Check sheet for the modelled part. Datum: model origin and axes. Units: mm. A direction names the side the tool comes from. Coordinates: 2 decimals unless noted, no trailing zeros. Loops run counter-clockwise (first coordinate to the right, second up) from the corner with the lowest first, then second, coordinate; pieces in that order, holes last. Notation, with made-up numbers: M 10.25,65.25 L 14.25,65.25 A14 ccw 14.25,72.25 Z; hole C 64,67.5 d2. An arc over 180 degrees is marked long. Write each question's results on one line, items separated by ' | '. Start each with the question number.
from build123d import *

# Parameters (mm, degrees)
F0_W      = 95
F0_H      = 138.5
F1_DEPTH  = 2.5
F2_W      = 95
F2_H      = 138.5
F2_W_2    = 62
F2_H_2    = 123
F3_DEPTH  = 8.5
F4_W      = 95
F4_H      = 138.5
F5_DEPTH  = 23.5
F6_W      = 62
F6_H      = 123
F7_DEPTH  = 23.501
F8_W      = 95
F8_H      = 138.5
F8_W_2    = 90
F8_H_2    = 133.5
F9_DEPTH  = 17.5
F11_ANGLE = 180
F13_ANGLE = 180
F14_W     = 0.75
F14_H     = 7.75
F16_W     = 0.75
F16_H     = 7.75


with BuildPart() as f1:
    # F0 (on Top) → F1 (new body)
    with BuildSketch(Plane.XY):
        Rectangle(F0_W, F0_H)
    extrude(amount=F1_DEPTH)

    # F2 (on face) → F3 (join)
    with BuildSketch(Plane.XY.offset(2.5)):
        Rectangle(F2_W, F2_H)
        Rectangle(F2_W_2, F2_H_2, mode=Mode.SUBTRACT)
    extrude(amount=F3_DEPTH)

    # F4 (on face) → F5 (join)
    with BuildSketch(Plane.XY.offset(11)):
        with BuildLine():
            ThreePointArc((-22.25, 22.25), (-6.516874, 28.766874), (0, 44.5))
            ThreePointArc((0, 44.5), (-37.983126, 60.233126), (-22.25, 22.25))
        make_face()
        with BuildLine():
            ThreePointArc((44.5, 44.5), (22.25, 66.75), (0, 44.5))
            ThreePointArc((0, 44.5), (6.516874, 28.766874), (22.25, 22.25))
            ThreePointArc((22.25, 22.25), (37.983126, 28.766874), (44.5, 44.5))
        make_face()
        with BuildLine():
            ThreePointArc((0, 0), (-6.516874, 15.733126), (-22.25, 22.25))
            ThreePointArc((-22.25, 22.25), (-44.5, 0), (-22.25, -22.25))
            ThreePointArc((-22.25, -22.25), (-6.516874, -15.733126), (0, 0))
        make_face()
        with BuildLine():
            ThreePointArc((44.5, 0), (37.983126, 15.733126), (22.25, 22.25))
            ThreePointArc((22.25, 22.25), (6.516874, 15.733126), (0, 0))
            ThreePointArc((0, 0), (6.516874, -15.733126), (22.25, -22.25))
            ThreePointArc((22.25, -22.25), (37.983126, -15.733126), (44.5, 0))
        make_face()
        with BuildLine():
            ThreePointArc((0, -44.5), (-6.516874, -28.766874), (-22.25, -22.25))
            ThreePointArc((-22.25, -22.25), (-37.983126, -60.233126), (0, -44.5))
        make_face()
        with BuildLine():
            ThreePointArc((44.5, -44.5), (37.983126, -28.766874), (22.25, -22.25))
            ThreePointArc((22.25, -22.25), (6.516874, -28.766874), (0, -44.5))
            ThreePointArc((0, -44.5), (22.25, -66.75), (44.5, -44.5))
        make_face()
        Rectangle(F4_W, F4_H)
        with BuildLine():
            ThreePointArc((-22.25, 22.25), (-37.983126, 60.233126), (0, 44.5))
            ThreePointArc((0, 44.5), (22.25, 66.75), (44.5, 44.5))
            ThreePointArc((44.5, 44.5), (37.983126, 28.766874), (22.25, 22.25))
            ThreePointArc((22.25, 22.25), (37.983126, 15.733126), (44.5, 0))
            ThreePointArc((44.5, 0), (37.983126, -15.733126), (22.25, -22.25))
            ThreePointArc((22.25, -22.25), (37.983126, -28.766874), (44.5, -44.5))
            ThreePointArc((44.5, -44.5), (22.25, -66.75), (0, -44.5))
            ThreePointArc((0, -44.5), (-37.983126, -60.233126), (-22.25, -22.25))
            ThreePointArc((-22.25, -22.25), (-44.5, 0), (-22.25, 22.25))
        make_face(mode=Mode.SUBTRACT)
    extrude(amount=F5_DEPTH)

    # F6 (on face) → F7 (cut, through all)
    with BuildSketch(Plane.XY.offset(11)):
        Rectangle(F6_W, F6_H)
    extrude(amount=F7_DEPTH, mode=Mode.SUBTRACT)

    # F8 (on face) → F9 (join)
    with BuildSketch(Plane.XY.offset(34.5)):
        Rectangle(F8_W, F8_H)
        Rectangle(F8_W_2, F8_H_2, mode=Mode.SUBTRACT)
    extrude(amount=F9_DEPTH)

    # F10 (on face) → F11 (revolve)
    with BuildSketch(Plane.YZ.offset(-45)):
        with BuildLine():
            Line((0, 36.5), (0, 34.5))
            ThreePointArc((0, 34.5), (1.414214, 35.085786), (2, 36.5))
            Line((2, 36.5), (2, 50))
            ThreePointArc((2, 50), (1.414214, 51.414214), (0, 52))
            Line((0, 52), (0, 50))
            Line((0, 50), (0, 36.5))
        make_face()
    revolve(axis=Axis((-45, 0, 43.25), (0, 0, -1)), revolution_arc=F11_ANGLE)

    # F12 (on face) → F13 (revolve)
    with BuildSketch(Plane(origin=(45, 0, 0), x_dir=(0, -1, 0), z_dir=(-1, 0, 0))):
        with BuildLine():
            ThreePointArc((-2, 36.5), (-1.414214, 35.085786), (0, 34.5))
            Line((0, 34.5), (0, 36.5))
            Line((0, 36.5), (0, 50))
            Line((0, 50), (-2, 50))
            Line((-2, 50), (-2, 36.5))
        make_face()
        with BuildLine():
            Line((-2, 50), (0, 50))
            Line((0, 50), (0, 52))
            ThreePointArc((0, 52), (-1.414214, 51.414214), (-2, 50))
        make_face()
    revolve(axis=Axis((45, 0, 43.25), (0, 0, 1)), revolution_arc=F13_ANGLE)

    # F14 (on face) → F15 (revolve)
    with BuildSketch(Plane.YZ.offset(-31)):
        with BuildLine():
            ThreePointArc((0.75, 10.25), (0.53033, 10.78033), (0, 11))
            Line((0, 11), (0, 10.25))
            Line((0, 10.25), (0.75, 10.25))
        make_face()
        with Locations((0.375, 6.375)):
            Rectangle(F14_W, F14_H)
    revolve(axis=Axis((-31, 0, 6.75), (0, 0, -1)))

    # F16 (on face) → F17 (revolve)
    with BuildSketch(Plane(origin=(31, 0, 0), x_dir=(0, -1, 0), z_dir=(-1, 0, 0))):
        with Locations((-0.375, 6.375)):
            Rectangle(F16_W, F16_H)
        with BuildLine():
            Line((-0.75, 10.25), (0, 10.25))
            Line((0, 10.25), (0, 11))
            ThreePointArc((0, 11), (-0.53033, 10.78033), (-0.75, 10.25))
        make_face()
    revolve(axis=Axis((31, 0, 6.75), (0, 0, 1)))


solid = f1.part
1) Set-up check for faces 5 (the flat face through (34, 49, 11)), 6 (the flat face through (47.5, -1, 26)): record each of +Z, -Z, +X, -X, +Y, -Y from which the full face is reachable in a straight line by a thin tool's end or side.
2) Section check A-A (z = 40). Enter the section's corners in (x, y), then the cut area to 3 significant figures.
3) Section check B-B (x = -36.5). Enter the section's corners in (y, z).
4) Gauge pin test, flat ends, axial feed: P1, Ø7, axis at x = -35, y = -10, coming from the +Z side; P2, Ø10, axis at x = -35, y = 22.5, coming from the +Z side; P3, Ø4, axis at x = 5.5, y = 5.5, coming from the +Z side. Record the tip position at first contact, or that the pin passes through.
5) Release check for a two-part mould opening along Y. For faces 1 (the flat face through (0, 67, 52)), 2 (the flat face through (-1, -69.25, 26)), 3 (the flat face through (-1, 69.25, 26)), 4 (the flat face through (0, 61.5, 15)) record: +Y half, -Y half, draft (parallel to the pull), parting line (faces both ways), or undercut.
6) Section check C-C (y = 49). Enter the section's corners in (x, z).
7) Thickness scan on probe 1 along Y at (x, z) = (28.5, 46); probe 2 along X at (y, z) = (-44.5, 21.25). Record the ranges inside material, lowest first.
8) Section check D-D (z = 22). Enter the section's corners in (x, y).
Return value:
1) face 5: +Z | face 6: +Z, -Z, +X, +Y, -Y
2) outline: M -47.5,-69.25 L 47.5,-69.25 L 47.5,69.25 L -47.5,69.25 Z; hole M -45,-66.75 L 45,-66.75 L 45,-2 A2 cw 45,2 L 45,66.75 L -45,66.75 L -45,2 A2 cw -45,-2 Z | area: 1,160 mm2
3) outline: M -69.25,0 L 69.25,0 L 69.25,52 L 66.75,52 L 66.75,34.5 L 61.59,34.5 L 61.59,11 L 27.41,11 L 27.41,34.5 L 17.09,34.5 L 17.09,11 L -17.09,11 L -17.09,34.5 L -27.41,34.5 L -27.41,11 L -61.59,11 L -61.59,34.5 L -66.75,34.5 L -66.75,52 L -69.25,52 Z
4) P1: stops at z = 11 | P2: stops at z = 34.5 | P3: stops at z = 2.5
5) face 1: draft | face 2: -Y half | face 3: +Y half | face 4: undercut
6) outline: M -47.5,0 L 47.5,0 L 47.5,52 L 45,52 L 45,34.5 L 44.04,34.5 L 44.04,11 L 31,11 L 31,2.5 L -31,2.5 L -31,11 L -44.04,11 L -44.04,34.5 L -45,34.5 L -45,52 L -47.5,52 Z
7) probe 1: y = -69.25 to -66.75, 66.75 to 69.25 | probe 2: x = -47.5 to -44.5, 44.5 to 47.5
8) outline: M -47.5,-69.25 L 47.5,-69.25 L 47.5,69.25 L -47.5,69.25 Z; hole M -31,-24.04 A22.25 ccw long -7.9,-61.5 L 7.9,-61.5 A22.25 ccw long 31,-24.04 L 31,-20.46 A22.25 ccw 31,20.46 L 31,24.04 A22.25 ccw long 7.9,61.5 L -7.9,61.5 A22.25 ccw long -31,24.04 L -31,20.46 A22.25 ccw -31,-20.46 Z
